Read the model definition and answer for the solid it produces. Units are mm, in the model's axes. Face numbers are marked on the shaded views. Coordinates: 2 decimals unless noted, no trailing zeros. Order: outer loops, then holes, each group sorted by start corner. A loop starts at its lowest first (then second) coordinate and runs counter-clockwise, first axis right, second up. Notation, with made-up numbers: M 39.5,37 L 73.5,37 A18 cw 73.5,68 Z; hole C 5,5 d5. An arc over 180 degrees is marked long. Use a Markdown table: item, result. Add a question column.
1) The mould has two halves that part along X. Classify the marked faces 1, 2, 3 and 4: released by +X, released by -X, zero draft, split by the parting line, or undercut.
2) Find section A-A on z = -14.5. Write down the section's boundary in (x, y).
3) Find section D-D on x = 24.5. Write down the section's boundary in (y, z).
4) Find the intervals of material crossed by probe 1 along Y at (x, z) = (-39, -33.02); probe 2 along X at (y, z) = (-9.5, -0.5); probe 3 along Z at (x, y) = (-2, -3.75), in increasing order. Write a range as [from, to].
5) Find section C-C on z = -23.5. Write down the section's boundary in (x, y), plus the area to 3 significant figures.
6) Find section B-B on y = -10.5. Write down the section's boundary in (x, z).
7) Each of these flat-tipped pins is pushed along its axis until it touches: pin 1 Ø8 at (y, z) = (-4, -4.5) entering from +X; pin 2 Ø1.3 at (y, z) = (-3.5, -1.5) entering from -X; pin 3 Ø5.5 at (x, y) = (0.5, -10.5) entering from -Z. Where does it stop, or does it pass through?
from build123d import *

# Parameters (mm, degrees)
F1_DEPTH      = 25.4
F3_DEPTH      = 40.641
F3_DEPTH_BACK = 40.641
F4_R          = 0.508
F5_DEPTH      = 40.641
F5_DEPTH_BACK = 40.641
F6_T1_DEPTH   = 17.4583858324
F6_T3_DEPTH   = 21.082
F6_T5_DEPTH   = 21.082
F6_T7_DEPTH   = 17.4583858324


# Not quite as in the source:
# - a fillet or chamfer that OpenCascade refuses, or shapes differently, is made with other operations: its cross-section is extruded or revolved along the edge and cut away or added


with BuildPart() as f1:
    # F0 (on Front) → F1 (new body)
    with BuildSketch(Plane.XZ):
        with BuildLine():
            Line((2.54, 0), (0, 0))
            Line((0, 0), (-2.54, 0))
            Line((-2.54, 0), (-14.478, 0))
            Line((-14.478, 0), (-17.018, 0))
            Line((-17.018, 0), (-17.018, -2.8580148686))
            ThreePointArc((-17.018, -2.8580148686), (-34.1882369177, -16.8868177776), (-40.64, -38.1))
            Line((-40.64, -38.1), (-38.608, -38.1))
            ThreePointArc((-38.608, -38.1), (-28.0439273838, -12.5960726162), (-2.54, -2.032))
            Line((-2.54, -2.032), (0, -2.032))
            Line((0, -2.032), (2.54, -2.032))
            ThreePointArc((2.54, -2.032), (28.0439273838, -12.5960726162), (38.608, -38.1))
            Line((38.608, -38.1), (40.64, -38.1))
            ThreePointArc((40.64, -38.1), (34.1882369177, -16.8868177776), (17.018, -2.8580148686))
            Line((17.018, -2.8580148686), (17.018, 0))
            Line((17.018, 0), (14.478, 0))
            Line((14.478, 0), (2.54, 0))
        make_face()
        Polygon((-17.018, 0), (-14.478, 0), (-17.018, 1.5875), align=None)
        Polygon((17.018, 1.5875), (14.478, 0), (17.018, 0), align=None)
    extrude(amount=F1_DEPTH)

    # F2 (on Right) → F3 (cut, two sides)
    with BuildSketch(Plane.YZ) as f3_sk:
        Polygon((-30.48, -50.8), (-3.4853166679, -50.8), (-30.48, 76.2), align=None)
    extrude(amount=-F3_DEPTH, mode=Mode.SUBTRACT)
    extrude(f3_sk.sketch, amount=F3_DEPTH_BACK, mode=Mode.SUBTRACT)

    # F4 (on Right) → F5 (cut, two sides)
    with BuildSketch(Plane.YZ) as f5_sk:
        with Locations((-3.81, -33.02)):
            Circle(F4_R)
    extrude(amount=-F5_DEPTH, mode=Mode.SUBTRACT)
    extrude(f5_sk.sketch, amount=F5_DEPTH_BACK, mode=Mode.SUBTRACT)

    # F6: fillet of radius 3.81 on 4 edges, made by hand

    # F6_s2 → F6_t1 (cut)
    with BuildSketch(Plane.YZ.offset(30.8948070838)):
        with BuildLine():
            ThreePointArc((-6.8262501934, -35.082143542), (-5.4972185245, -37.2509261132), (-3.0995078346, -38.1))
            Line((-3.0995078346, -38.1), (-6.1847850011, -38.1))
            Line((-6.1847850011, -38.1), (-6.8262501934, -35.082143542))
        make_face()
    extrude(amount=F6_T1_DEPTH, mode=Mode.SUBTRACT)

    # F6_s4 → F6_t3 (cut)
    with BuildSketch(Plane.YZ.offset(29.083)):
        with BuildLine():
            ThreePointArc((0, -34.29), (-1.1159231637, -36.9840768363), (-3.81, -38.1))
            Line((-3.81, -38.1), (0, -38.1))
            Line((0, -38.1), (0, -34.29))
        make_face()
    extrude(amount=F6_T3_DEPTH, mode=Mode.SUBTRACT)

    # F6_s6 → F6_t5 (cut)
    with BuildSketch(Plane.YZ.offset(-50.165)):
        with BuildLine():
            ThreePointArc((0, -34.29), (-1.1159231637, -36.9840768363), (-3.81, -38.1))
            Line((-3.81, -38.1), (0, -38.1))
            Line((0, -38.1), (0, -34.29))
        make_face()
    extrude(amount=F6_T5_DEPTH, mode=Mode.SUBTRACT)

    # F6_s8 → F6_t7 (cut)
    with BuildSketch(Plane.YZ.offset(-48.3531929162)):
        with BuildLine():
            ThreePointArc((-6.8262501934, -35.082143542), (-5.4972185245, -37.2509261132), (-3.0995078346, -38.1))
            Line((-3.0995078346, -38.1), (-6.1847850011, -38.1))
            Line((-6.1847850011, -38.1), (-6.8262501934, -35.082143542))
        make_face()
    extrude(amount=F6_T7_DEPTH, mode=Mode.SUBTRACT)


solid = f1.part
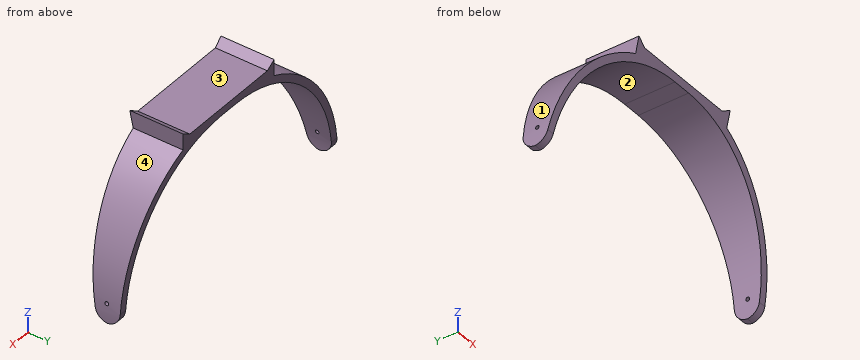
Check result:
| question | item | result |
|---|---|---|
| 1 | face 1 | released by -X |
| 1 | face 2 | undercut |
| 1 | face 3 | undercut |
| 1 | face 4 | released by +X |
| 2 | outline | M -32.45,-11.2 L -29.82,-11.2 L -29.82,0 L -32.45,0 Z; M 29.82,-11.2 L 32.45,-11.2 L 32.45,0 L 29.82,0 Z |
| 3 | outline | M -12.8,-6.97 L -12.27,-9.49 L 0,-9.49 L 0,-6.97 Z |
| 4 | probe 1 | y = [-7.26, -4.32], [-3.3, 0] |
| 4 | probe 2 | x = [-17.02, 17.02] |
| 4 | probe 3 | z = [-2.03, 0] |
| 5 | outline | M -37.73,-9.29 L -35.52,-9.29 L -35.52,0 L -37.73,0 Z; M 35.52,-9.29 L 37.73,-9.29 L 37.73,0 L 35.52,0 Z |
| 5 | area | 41.1 mm2 |
| 6 | outline | M -34.78,-17.8 L -32.35,-17.8 A36.07 cw -2.54,-2.03 L 2.54,-2.03 A36.07 cw 32.35,-17.8 L 34.78,-17.8 A38.1 ccw 17.02,-2.86 L 17.02,1.59 L 14.48,0 L -14.48,0 L -17.02,1.59 L -17.02,-2.86 A38.1 ccw Z |
| 7 | pin 1 | stops at x = 26.53 |
| 7 | pin 2 | stops at x = -17.02 |
| 7 | pin 3 | stops at z = -2.04 |
